Can you work these out from the drawing? Everything is in mm from the part's minimum corner. Round coordinates to 2 decimals unless told otherwise and drop trailing zeros. Loops run counter-clockwise (first coordinate to the right, second up) from the corner with the lowest first, then second, coordinate; pieces in that order, holes last. Notation, with made-up numbers: (52.25, 82) -> (81.25, 82) arc R14 ccw to (81.25, 106) -> close; hole circle Ø2 at (77, 44). An arc over 180 degrees is marked (long way). One line per item, written item: value.
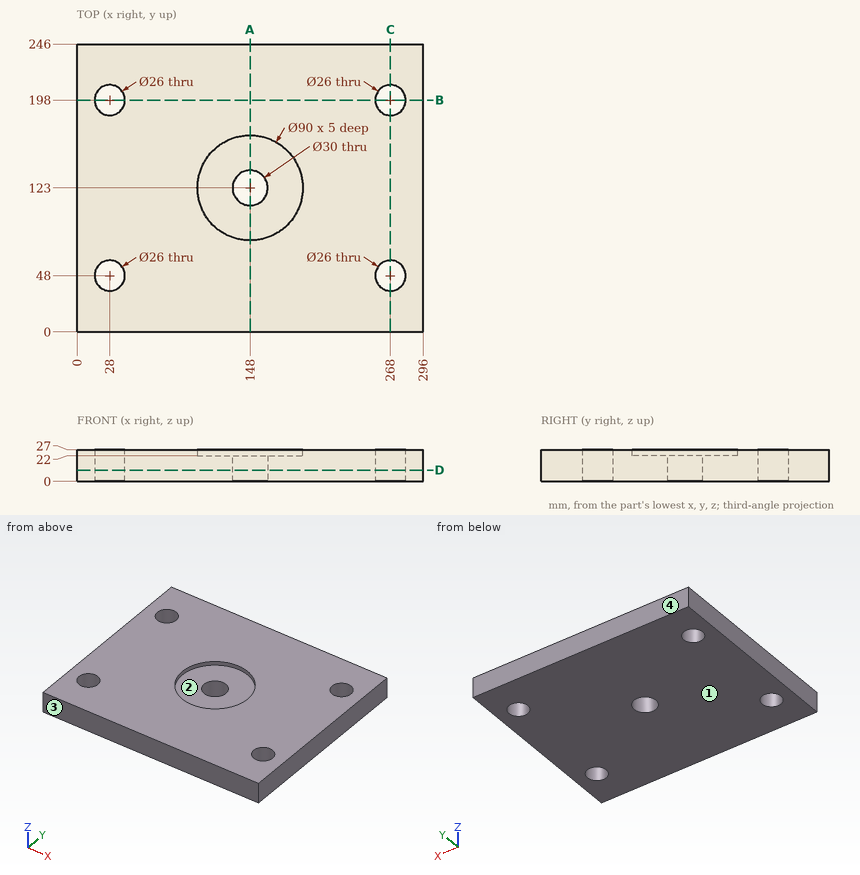
(1) For pin 1 Ø3 at (x, y) = (160, 210) entering from -Z; pin 2 Ø23.5 at (x, y) = (268, 198) entering from +Z, each with a flat end and sliding along its axis, tell me the tip position at first contact or that it passes through.
Results below:
pin 1: stops at z = 0
pin 2: passes through
(2) We'd pull the mould along Y, two halves only. Please class the marked faces 1, 2, 3 and 4: +Y half, -Y half, draft (parallel to the pull), parting line (faces both ways), or undercut.
Results below:
face 1: draft
face 2: undercut
face 3: -Y half
face 4: +Y half
(3) Imagine slicing it at A-A on x = 148. Write out the boundary of the cut face in (y, z).
Results below:
outline: (0, 0) -> (108, 0) -> (108, 22) -> (78, 22) -> (78, 27) -> (0, 27) -> close; (138, 0) -> (246, 0) -> (246, 27) -> (168, 27) -> (168, 22) -> (138, 22) -> close
(4) Please list where these lines run through material, in increasing order: L1, parallel to Y at x = 268, z = 20; L2, parallel to Y at x = 148, z = 6.5; L3, parallel to Y at x = 272.5, z = 2.5.
Results below:
L1: y = 0 to 35, 61 to 185, 211 to 246
L2: y = 0 to 108, 138 to 246
L3: y = 0 to 35.8, 60.2 to 185.8, 210.2 to 246
(5) Imagine slicing it at C-C on x = 268. Write out the boundary of the cut face in (y, z).
Results below:
outline: (0, 0) -> (35, 0) -> (35, 27) -> (0, 27) -> close; (61, 0) -> (185, 0) -> (185, 27) -> (61, 27) -> close; (211, 0) -> (246, 0) -> (246, 27) -> (211, 27) -> close
(6) Imagine slicing it at B-B on y = 198. Write out the boundary of the cut face in (x, z).
Results below:
outline: (0, 0) -> (15, 0) -> (15, 27) -> (0, 27) -> close; (41, 0) -> (255, 0) -> (255, 27) -> (41, 27) -> close; (281, 0) -> (296, 0) -> (296, 27) -> (281, 27) -> close
(7) Imagine slicing it at D-D on z = 9.5. Write out the boundary of the cut face in (x, y).
Results below:
outline: (0, 0) -> (296, 0) -> (296, 246) -> (0, 246) -> close; hole circle Ø26 at (28, 48); hole circle Ø26 at (28, 198); hole circle Ø30 at (148, 123); hole circle Ø26 at (268, 48); hole circle Ø26 at (268, 198)
